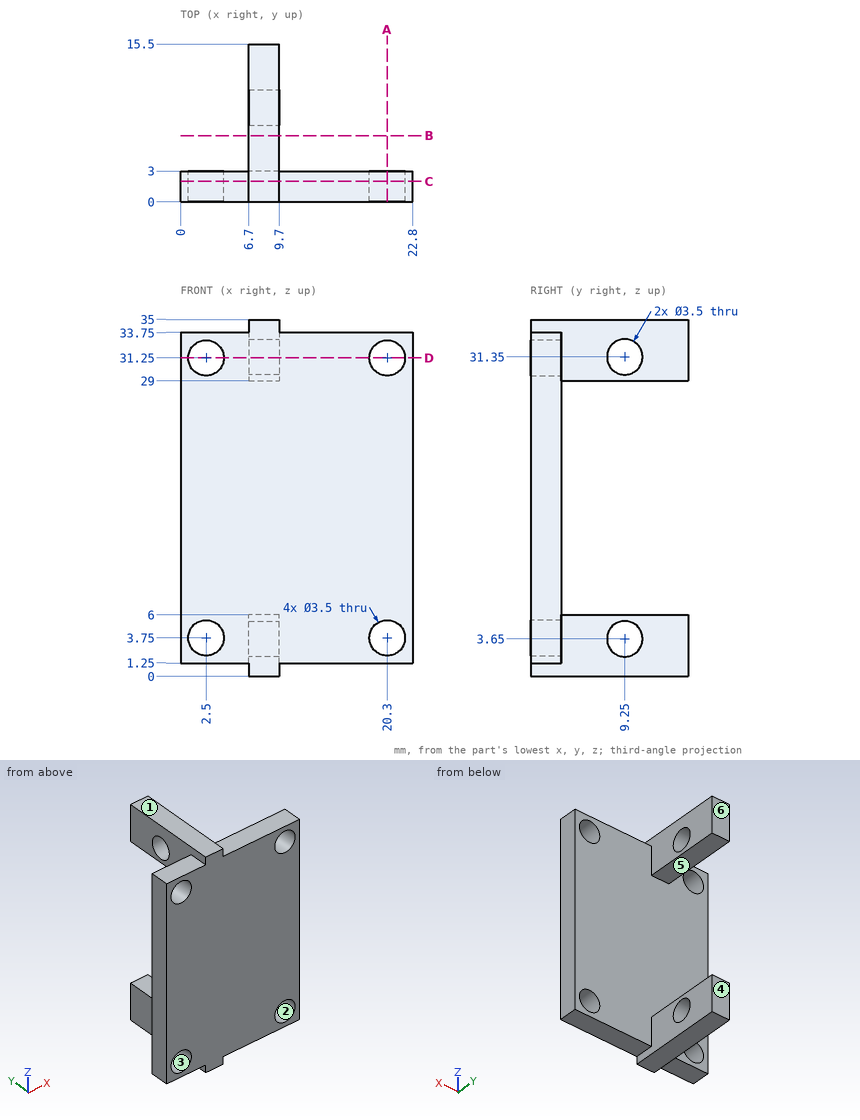
Part print with two shaded views. Sizes in mm from the minimum x, y, z corner. A direction names the side the tool comes from. Coordinates: 2 decimals unless noted, no trailing zeros. Write each loop counter-clockwise with the first axis right and the second up, starting at its lowest first coordinate (ties: lowest second). Pieces come first, ordered by that corner, then holes. Notation, with made-up numbers: (16.5, 53.25) - (28.5, 53.25) arc R20 cw to (28.5, 63.25) - close; hole circle Ø1 at (41, 77.5). An arc over 180 degrees is marked (long way). One line per item, written item: value. Start each with the question number.
1. Slice it at C-C (y = 2). Write the cut outline in (x, z), plus the area to 3 significant figures.
2. Slice it at D-D (z = 31.25). Write the cut outline in (x, y).
3. Flat gauge pins, fed straight in: pin 1 (3.5 mm diameter, centred on x = 19, y = 1, fed in from -Z); pin 2 (8 mm diameter, centred on y = 10, z = 31, fed in from -X); pin 3 (3.5 mm diameter, centred on x = 3, y = 1.5, fed in from +Z). Where does each tip first touch, or does it go through?
4. Slice it at B-B (y = 6.5). Write the cut outline in (x, z).
5. Tool access for the marked faces 5 and 6: list every direction of +Z, -Z, +X, -X, +Y, -Y with a clear straight run to the whole face (end or side of a thin tool).
6. Probe line 1 (Y direction, x = 8.75, z = 31.35); line 2 (Z direction, x = 8, y = 8.75); line 3 (X direction, y = 2.25, z = 31.5). List the from-to ranges inside material, lowest first. Write a range as from..to.
7. Slice it at A-A (x = 20.3). Write the cut outline in (y, z), plus the area to 3 significant figures.
8. Mould opens along Z. For the marked faces 1, 2, 3 and 4 say: released by +Z, released by -Z, zero draft, split by the parting line, or undercut.
Answers below:
1. outline: (0, 1.25) - (6.7, 1.25) - (6.7, 0) - (9.7, 0) - (9.7, 1.25) - (22.8, 1.25) - (22.8, 33.75) - (9.7, 33.75) - (9.7, 35) - (6.7, 35) - (6.7, 33.75) - (0, 33.75) - close; hole circle Ø3.5 at (2.5, 3.75); hole circle Ø3.5 at (2.5, 31.25); hole circle Ø3.5 at (20.3, 3.75); hole circle Ø3.5 at (20.3, 31.25)
1. area: 710 mm^2
2. outline: (0, 0) - (0.75, 0) - (0.75, 3) - (0, 3) - close; (4.25, 0) - (18.55, 0) - (18.55, 3) - (9.7, 3) - (9.7, 7.5) - (6.7, 7.5) - (6.7, 3) - (4.25, 3) - close; (6.7, 11) - (9.7, 11) - (9.7, 15.5) - (6.7, 15.5) - close; (22.05, 0) - (22.8, 0) - (22.8, 3) - (22.05, 3) - close
3. pin 1: stops at z = 1.25
3. pin 2: stops at x = 6.7
3. pin 3: stops at z = 33.75
4. outline: (6.7, 0) - (9.7, 0) - (9.7, 6) - (6.7, 6) - close; (6.7, 29) - (9.7, 29) - (9.7, 35) - (6.7, 35) - close
5. face 5: +X, -X, +Y
5. face 6: +Z, -Z, +X, -X, +Y
6. line 1: y = 0..7.5, 11..15.5
6. line 2: z = 0..1.97, 5.33..6, 29..29.67, 33.03..35
6. line 3: x = 0..0.77, 4.23..18.57, 22.03..22.8
7. outline: (0, 1.25) - (3, 1.25) - (3, 2) - (0, 2) - close; (0, 5.5) - (3, 5.5) - (3, 29.5) - (0, 29.5) - close; (0, 33) - (3, 33) - (3, 33.75) - (0, 33.75) - close
7. area: 76.5 mm^2
8. face 1: released by +Z
8. face 2: undercut
8. face 3: undercut
8. face 4: zero draft
